Here's how the part is built. I have some questions about the finished solid (model axes, mm). A direction names the side the tool comes from. Give positions to 0.01 mm unless a question says otherwise; leave off trailing zeros. Write each loop counter-clockwise with the first axis right and the second up, starting at its lowest first coordinate (ties: lowest second). Pieces come first, ordered by that corner, then holes. Notation, with made-up numbers: (40.25, 70.25) -> (92.25, 70.25) arc R25 cw to (92.25, 90.25) -> close; hole circle Ø8 at (82.25, 23.5). An arc over 180 degrees is marked (long way). Use one line per item in the form item = value.
```python
from build123d import *

# Parameters (mm, degrees)
SKETCH4_W           = 6
SKETCH4_H           = 2
BOSS_EXTRUDE3_DEPTH = 0.4
SKETCH6_R           = 0.75
BOSS_EXTRUDE4_DEPTH = 4.5


with BuildPart() as part:
    # Sketch4 → Boss-Extrude3 (new body)
    with BuildSketch(Plane.XY.offset(5)):
        with Locations((-1, 0)):
            Rectangle(SKETCH4_W, SKETCH4_H)
    extrude(amount=BOSS_EXTRUDE3_DEPTH)

    # Sketch6 → Boss-Extrude4 (add)
    with BuildSketch(Plane.XY.offset(5)):
        Circle(SKETCH6_R)
    extrude(amount=-BOSS_EXTRUDE4_DEPTH)


solid = part.part
```
Q1. Will these pins go through, and if not, where does the flat tip stop? pin 1 Ø2 at (x, z) = (-0.5, 3.5) entering from +Y; pin 2 Ø0.6 at (x, y) = (-2, -0.5) entering from -Z.
Result set:
pin_1 = 0.75
pin_2 = 5
Q2. I want a section at C-C, the plane z = 2. Write out the boundary of the cut face in (x, y).
Result set:
outline = circle Ø1.5 at (0, 0)
Q3. I want a section at D-D, the plane x = -3.6. Write out the boundary of the cut face in (y, z), and give its area (3 significant figures).
Result set:
outline = (-1, 5) -> (1, 5) -> (1, 5.4) -> (-1, 5.4) -> close
area = 0.800 mm2
Q4. I want a section at A-A, the plane x = 0. Write out the boundary of the cut face in (y, z).
Result set:
outline = (-1, 5) -> (-0.75, 5) -> (-0.75, 0.5) -> (0.75, 0.5) -> (0.75, 5) -> (1, 5) -> (1, 5.4) -> (-1, 5.4) -> close
Q5. Which directions (+Z, -Z, +X, -X, +Y, -Y) give clear straight access to the entire face, cutting with the end or side of a thin tool? Please do faces 1 (the face through (-1, 0, 5.4)), 2 (the face through (-0.75, 0.03, 2.78)).
Result set:
face_1 = +Z, +X, -X, +Y, -Y
face_2 = -Z
Q6. I want a section at B-B, the plane y = -0.3. Write out the boundary of the cut face in (x, z), and give its area (3 significant figures).
Result set:
outline = (-4, 5) -> (-0.69, 5) -> (-0.69, 0.5) -> (0.69, 0.5) -> (0.69, 5) -> (2, 5) -> (2, 5.4) -> (-4, 5.4) -> close
area = 8.59 mm2
Q7. If I drill on line 1 along Z through (x, y) = (-1.05, -0.4); line 2 along X through (y, z) = (0.05, 3.65), over which ranges is the centre line in solid material (lowest first)? Write a range as from..to.
Result set:
line_1 = 5..5.4
line_2 = -0.75..0.75
